Part model, mm, in its own coordinate system. A direction names the side the tool comes from. Round coordinates to 2 decimals unless told otherwise and drop trailing zeros. Loops run counter-clockwise (first coordinate to the right, second up) from the corner with the lowest first, then second, coordinate; pieces in that order, holes last.
1) Mould opens along Y. For faces 1 (the flat face through (6, 0, 288)), 2 (the flat face through (12, 6, 0)), 3 (the flat face through (6, 1.588, 288)) say: +Y half, -Y half, draft (parallel to the pull), parting line (faces both ways), or undercut.
2) Band-saw the part on A-A, the plane x = 6.35. Write the cut outline in (y, z).
3) Drop a flat-ended pin along its axis: P1, Ø4.5, axis at x = 6.35, z = 25.4, coming from the -Y side. Give the stop position or say it passes through.
4) Probe line 1 (X direction, y = 8, z = 549); line 2 (Z direction, x = 6.35, y = 11.7). List the from-to ranges inside material, lowest first.
5) Band-saw the part on B-B, the plane z = 242.5. Write the cut outline in (x, y).
6) 3-axis set-ups, long thin cutter, end or side, ignore diameter. For faces 4 (the flat face through (6, 12.7, 288)), 5 (the flat face through (1.588, 6, 288)): which of +Z, -Z, +X, -X, +Y, -Y reach the whole face in a straight line?
Autodesk Inventor part; units mm, degrees
ref_plane "YZ Plane" through (0, 0, 0) normal (1, 0, 0) x (0, 1, 0)
ref_plane "XZ Plane" through (0, 0, 0) normal (0, 1, 0) x (-1, 0, 0)
ref_plane "XY Plane" through (0, 0, 0) normal (0, 0, 1) x (1, 0, 0)
sketch "Sketch1" plane through (0, 0, 0) normal (0, 0, 1) x (1, 0, 0)
  line L0 (0, 0) -> (12.7, 0)
  line L1 (12.7, 0) -> (12.7, 12.7)
  line L2 (12.7, 12.7) -> (0, 12.7)
  line L3 (0, 12.7) -> (0, 0)
  dimension "d0" = 12.7
  dimension "d1" = 12.7
extrude "Extrusion1" add sketch "Sketch1" along normal blind 584.2
shell "Shell1" thickness 1.5875 removed faces 2 at (8.4667, 8.4667, 0) at (8.4667, 8.4667, 584.2)
sketch "Sketch2" plane through (0, 0, 0) normal (0, -1, 0) x (1, 0, 0)
  line L0 (0, 0) -> (0, 584.2)
  line L1 (0, 0) -> (12.7, 0)
  circle A0 centre (6.35, 25.4) radius 2.4384
  dimension "d5" = 4.8768
  dimension "d6" = 6.35
  dimension "d7" = 25.4
extrude "Extrusion2" cut sketch "Sketch2" against normal through all
properties part number "Shovel_RollerAxle" material "Aluminum-6061"
Reported:
1. face 1: -Y half
1. face 2: draft
1. face 3: undercut
2. outline: (0, 0) - (1.59, 0) - (1.59, 22.96) - (0, 22.96) - close; (0, 27.84) - (1.59, 27.84) - (1.59, 584.2) - (0, 584.2) - close; (11.11, 0) - (12.7, 0) - (12.7, 22.96) - (11.11, 22.96) - close; (11.11, 27.84) - (12.7, 27.84) - (12.7, 584.2) - (11.11, 584.2) - close
3. P1: passes through
4. line 1: x = 0 to 1.59, 11.11 to 12.7
4. line 2: z = 0 to 22.96, 27.84 to 584.2
5. outline: (0, 0) - (12.7, 0) - (12.7, 12.7) - (0, 12.7) - close; hole (1.59, 1.59) - (11.11, 1.59) - (11.11, 11.11) - (1.59, 11.11) - close
6. face 4: +Z, -Z, +X, -X, +Y
6. face 5: +Z, -Z
